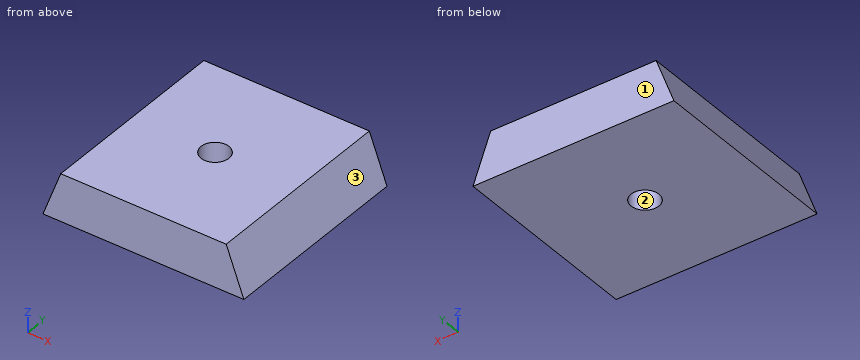
from build123d import *

# Parameters (mm, degrees)
F0_W     = 34
F0_H     = 33
F0_R     = 2.366828
F1_DEPTH = 8
F3_DEPTH = 35


with BuildPart() as f1:
    # F0 (on Top) → F1 (new body)
    with BuildSketch(Plane.XY):
        Rectangle(F0_W, F0_H)
        Circle(F0_R, mode=Mode.SUBTRACT)
    extrude(amount=F1_DEPTH)

    # F2 (on face) → F3 (cut)
    with BuildSketch(Plane.XZ.offset(16.5)):
        Polygon((-17, 0), (-13.995684, 8), (-17, 8), align=None)
        Polygon((17, 8), (14.007485, 8), (17, 0), align=None)
    extrude(amount=-F3_DEPTH, mode=Mode.SUBTRACT)


solid = f1.part
Could you check a few things on this model? Use its own coordinates, in mm. Face numbers are marked on the shaded views. Round coordinates to 2 decimals unless told otherwise and drop trailing zeros. Order: outer loops, then holes, each group sorted by start corner. A loop starts at its lowest first (then second) coordinate and runs counter-clockwise, first axis right, second up.
Q1. Imagine slicing it at C-C, the plane z = 4.25. List the corners of the cut face in (x, y) for me, then the cut area to 3 significant figures.
Geometry says:
outline: (-15.4, -16.5) - (15.41, -16.5) - (15.41, 16.5) - (-15.4, 16.5) - close; hole circle Ø4.73 at (0, 0)
area: 999 mm2
Q2. Please list where these lines run through material, in increasing order: probe 1 along Y at (x, z) = (0, 4); probe 2 along X at (y, z) = (-11, 3.5); probe 3 along X at (y, z) = (-1, 1).
Geometry says:
probe 1: y = -16.5 to -2.37, 2.37 to 16.5
probe 2: x = -15.69 to 15.69
probe 3: x = -16.62 to -2.15, 2.15 to 16.63
Q3. Imagine slicing it at B-B, the plane x = 0. List the corners of the cut face in (y, z) for me.
Geometry says:
outline: (-16.5, 0) - (-2.37, 0) - (-2.37, 8) - (-16.5, 8) - close; (2.37, 0) - (16.5, 0) - (16.5, 8) - (2.37, 8) - close
Q4. Imagine slicing it at A-A, the plane y = 0. List the corners of the cut face in (x, z) for me, then the cut area to 3 significant figures.
Geometry says:
outline: (-17, 0) - (-2.37, 0) - (-2.37, 8) - (-14, 8) - close; (2.37, 0) - (17, 0) - (14.01, 8) - (2.37, 8) - close
area: 210 mm2
Q5. Imagine slicing it at D-D, the plane y = -11. List the corners of the cut face in (x, z) for me, then the cut area to 3 significant figures.
Geometry says:
outline: (-17, 0) - (17, 0) - (14.01, 8) - (-14, 8) - close
area: 248 mm2
Q6. Thinking about a two-plate mould opening in Y: for the marked faces 1, 2 and 3, which applies, released by +Y, released by -Y, zero draft, split by the parting line, or undercut?
Geometry says:
face 1: released by +Y
face 2: undercut
face 3: zero draft
